Source: three-view drawing plus pictorial views. Frame: mm from the lowest corner of the part. A direction names the side the tool comes from. Give positions to 0.01 mm unless a question says otherwise; leave off trailing zeros. Write each loop counter-clockwise with the first axis right and the second up, starting at its lowest first coordinate (ties: lowest second). Pieces come first, ordered by that corner, then holes. Notation, with made-up numbers: (46, -39) -> (89, -39) arc R31 cw to (89, -10) -> close; hole circle Ø2 at (-4.75, 27.25). An arc over 180 degrees is marked (long way). Answer in a Markdown table with one row per item. Add a question column.
Item 1: Section query B-B on z = 14.25. Output: boundary loops of the cut face in (x, y) (3 decimals).
Item 2: Draft query along X for the marked faces 1, 2 and 3. Return one class per face: +X half, -X half, draft (parallel to the pull), parting line (faces both ways), or undercut.
Item 3: Material intervals for probe 1 along X at (y, z) = (14.5, 4.5) (3 decimals); probe 2 along Y at (x, z) = (48.5, 9.5) (3 decimals); probe 3 along X at (y, z) = (32.5, 11), sorted ascending. Write a range as from..to.
Item 4: Access query for the marked faces 4, 5 and 6. Directions: +Z, -Z, +X, -X, +Y, -Y. A direction counts if a zero-diameter tool reaches every point of the face in a straight line with its end or side. Return the directions, or none.
Item 5: Section query D-D on x = 83.5. Output: boundary loops of the cut face in (y, z) (3 decimals), plus the area to 3 significant figures.
Item 6: Section query C-C on y = 29. Output: boundary loops of the cut face in (x, z).
Item 7: Section query A-A on y = 10. Output: boundary loops of the cut face in (x, z) (3 decimals).
Item 8: First-contact query: P1, Ø1, axis at y = 24, z = 15.5, coming from the +X side; P2, Ø1.5, axis at y = 26, z = 5, coming from the -X side; P3, Ø5, axis at x = 68, z = 12.5, coming from the -Y side. Flat tips, straight axial feed; report the tip coordinate or a pass-through.
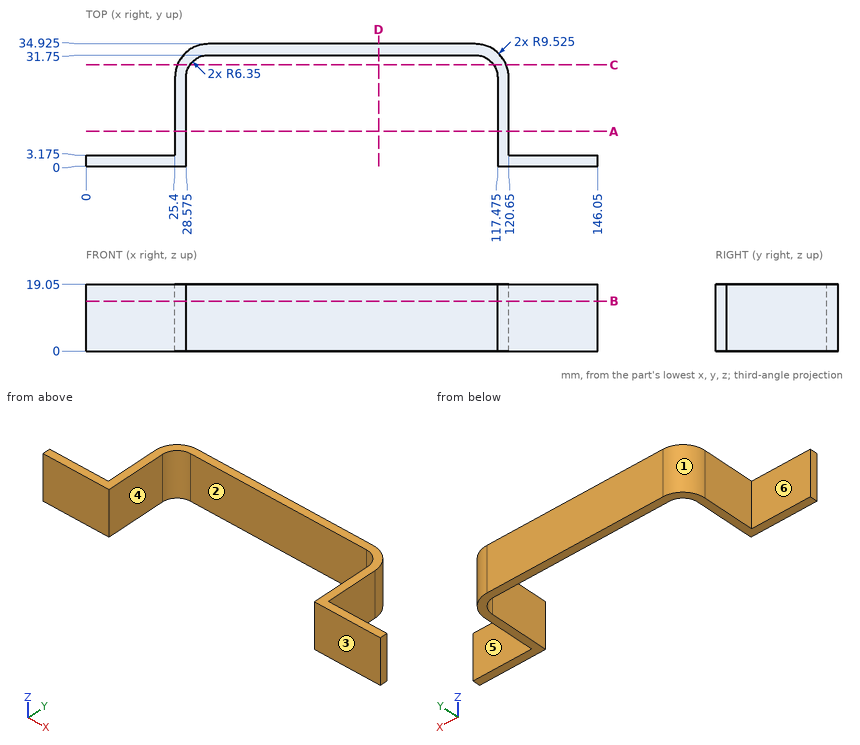
Findings below:
| question | item | result |
|---|---|---|
| 1 | outline | (0, 0) -> (28.575, 0) -> (28.575, 25.4) arc R6.35 cw to (34.925, 31.75) -> (111.125, 31.75) arc R6.35 cw to (117.475, 25.4) -> (117.475, 0) -> (146.05, 0) -> (146.05, 3.175) -> (120.65, 3.175) -> (120.65, 25.4) arc R9.525 ccw to (111.125, 34.925) -> (34.925, 34.925) arc R9.525 ccw to (25.4, 25.4) -> (25.4, 3.175) -> (0, 3.175) -> close |
| 2 | face 1 | -X half |
| 2 | face 2 | undercut |
| 2 | face 3 | draft |
| 3 | probe 1 | x = 25.4..28.575, 117.475..120.65 |
| 3 | probe 2 | y = 31.75..34.925 |
| 3 | probe 3 | x = 28.58..117.47 |
| 4 | face 4 | +Z, -Z, -Y |
| 4 | face 5 | +Z, -Z, +X, +Y |
| 4 | face 6 | +Z, -Z, -X, +Y |
| 5 | outline | (31.75, 0) -> (34.925, 0) -> (34.925, 19.05) -> (31.75, 19.05) -> close |
| 5 | area | 60.5 mm^2 |
| 6 | outline | (26.11, 0) -> (29.69, 0) -> (29.69, 19.05) -> (26.11, 19.05) -> close; (116.36, 0) -> (119.94, 0) -> (119.94, 19.05) -> (116.36, 19.05) -> close |
| 7 | outline | (25.4, 0) -> (28.575, 0) -> (28.575, 19.05) -> (25.4, 19.05) -> close; (117.475, 0) -> (120.65, 0) -> (120.65, 19.05) -> (117.475, 19.05) -> close |
| 8 | P1 | stops at x = 120.65 |
| 8 | P2 | stops at x = 25.4 |
| 8 | P3 | stops at y = 31.75 |
